```python
from build123d import *

# Parameters (mm, degrees)
F6_DEPTH = 22.5
F7_DEPTH = 2
F8_SIZE  = 2


with BuildPart() as f6:
    # F5 (on Right) → F6 (new body)
    with BuildSketch(Plane.YZ):
        Polygon((45.25, 2), (45.25, 0), (57.75, 0), (62.75, 0), (105.25, 0), (105.25, 2), (105.25, 17), (105.25, 19), (88.25, 19), (88.25, 17), (103.25, 17), (103.25, 2), align=None)
    extrude(amount=F6_DEPTH)

    # F4 (on Top) → F7 (cut, through all)
    with BuildSketch(Plane.XY):
        with BuildLine():
            ThreePointArc((18.25, 60.25), (17.517766953, 62.017766953), (15.75, 62.75))
            ThreePointArc((15.75, 62.75), (13.25, 60.25), (15.75, 57.75))
            ThreePointArc((15.75, 57.75), (17.517766953, 58.482233047), (18.25, 60.25))
        make_face()
        with BuildLine():
            ThreePointArc((5.5, 62.75), (7.267766953, 62.017766953), (8, 60.25))
            ThreePointArc((8, 60.25), (7.267766953, 58.482233047), (5.5, 57.75))
            Line((5.5, 57.75), (15.75, 57.75))
            ThreePointArc((15.75, 57.75), (13.25, 60.25), (15.75, 62.75))
            Line((15.75, 62.75), (5.5, 62.75))
        make_face()
        with BuildLine():
            ThreePointArc((5.5, 57.75), (7.267766953, 58.482233047), (8, 60.25))
            ThreePointArc((8, 60.25), (7.267766953, 62.017766953), (5.5, 62.75))
            ThreePointArc((5.5, 62.75), (3, 60.25), (5.5, 57.75))
        make_face()
    extrude(amount=F7_DEPTH, mode=Mode.SUBTRACT)

    # F8
    f8_edges = [f6.edges().sort_by_distance(p)[0] for p in [
        (11.25, 103.25, 2),
        (11.25, 103.25, 17),
    ]]
    chamfer(f8_edges, length=F8_SIZE)


solid = f6.part
```
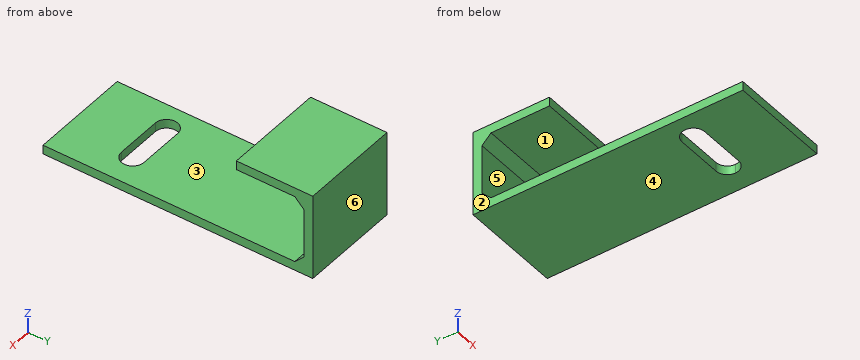
CAD build for the part. Positions are in the model's coordinates, mm. Face numbers are marked on the shaded views. A direction names the side the tool comes from. Give positions to 0.01 mm unless a question says otherwise; leave off trailing zeros. Write each loop counter-clockwise with the first axis right and the second up, starting at its lowest first coordinate (ties: lowest second). Pieces come first, ordered by that corner, then holes. Notation, with made-up numbers: (12, 50.5) -> (31, 50.5) arc R24 ccw to (31, 74.5) -> close; hole circle Ø9 at (56.25, -38.75). An arc over 180 degrees is marked (long way). Write each question's results on one line, items separated by ' | '.
1. Cut at A-A, the plane x = 6.5. Write the cut outline in (y, z).
Geometry check:
outline: (45.25, 0) -> (57.75, 0) -> (57.75, 2) -> (45.25, 2) -> close; (62.75, 0) -> (105.25, 0) -> (105.25, 19) -> (88.25, 19) -> (88.25, 17) -> (101.25, 17) -> (103.25, 15) -> (103.25, 4) -> (101.25, 2) -> (62.75, 2) -> close
2. Drop flat-ended pins along their axis: P1, Ø5.5, axis at x = 15, z = 11.5, coming from the -Y side; P2, Ø2, axis at x = 8.5, z = 18, coming from the -Y side. Give the stop position or say it passes through.
Geometry check:
P1: y = 103.25 | P2: y = 88.25
3. Wall check: probe 1 along Z at (x, y) = (1, 90.5); probe 2 along Y at (x, z) = (7.5, 1.25); probe 3 along Z at (x, y) = (11, 85.5). Give the ranges that are in metal, low to high. Write a range as [from, to].
Geometry check:
probe 1: [0, 2], [17, 19] | probe 2: [45.25, 57.75], [62.75, 105.25] | probe 3: [0, 2]
4. Cut at C-C, the plane x = 20.5. Write the cut outline in (y, z).
Geometry check:
outline: (45.25, 0) -> (105.25, 0) -> (105.25, 19) -> (88.25, 19) -> (88.25, 17) -> (101.25, 17) -> (103.25, 15) -> (103.25, 4) -> (101.25, 2) -> (45.25, 2) -> close
5. Two-plate mould, pull along Z, no slides. Class the marked faces 3, 4, 5 and 6: pulls with the +Z half, pulls with the -Z half, needs draft (parallel to the pull), parting line crosses it, or undercut.
Geometry check:
face 3: undercut | face 4: pulls with the -Z half | face 5: undercut | face 6: needs draft
6. Which spindle directions (+Z, -Z, +X, -X, +Y, -Y) get a long thin tool onto all of the face, cutting with end or side? Do the marked faces 1 and 2. Say none if no direction does.
Geometry check:
face 1: +X, -X, -Y | face 2: +Z, -Z, -X, +Y, -Y
7. Cut at D-D, the plane y = 62. Write the cut outline in (x, z).
Geometry check:
outline: (0, 0) -> (3.71, 0) -> (3.71, 2) -> (0, 2) -> close; (17.54, 0) -> (22.5, 0) -> (22.5, 2) -> (17.54, 2) -> close
8. Cut at B-B, the plane y = 100.5. Write the cut outline in (x, z), then the cut area to 3 significant figures.
Geometry check:
outline: (0, 0) -> (22.5, 0) -> (22.5, 2) -> (0, 2) -> close; (0, 17) -> (22.5, 17) -> (22.5, 19) -> (0, 19) -> close | area: 90.0 mm²
